from build123d import *

# Parameters (mm, degrees)
EXTRUDE_1_DEPTH     = 3
SKETCH_2_W          = 3
SKETCH_2_H          = 26
EXTRUDE_2_DEPTH     = 53.5
FILLET_1_R          = 4
FILLET_2_R          = 2
FILLET_3_R          = 1
SKETCH_3_W          = 1.7
SKETCH_3_H          = 1.7
CUT_EXTRUDE_1_DEPTH = 3
SKETCH_4_R          = 2
CUT_EXTRUDE_2_DEPTH = 1.6
SKETCH_5_W          = 1.7
SKETCH_5_H          = 1.7
CUT_EXTRUDE_3_DEPTH = 3
SKETCH_6_R          = 2
CUT_EXTRUDE_4_DEPTH = 1.6
CUT_EXTRUDE_5_DEPTH = 3


with BuildPart() as part:
    # Эскиз1 → Бобышка-Вытянуть1 (new body)
    with BuildSketch(Plane(origin=(0, 0, 0), x_dir=(1, 0, 0), z_dir=(0, 1, 0))):
        with BuildLine():
            Line((-27.082461997, 18.034885268), (36.497538003, 18.034885268))
            Line((36.497538003, 18.034885268), (36.497538003, -7.965114732))
            Line((36.497538003, -7.965114732), (-27.082461997, -7.965114732))
            ThreePointArc((-27.082461997, -7.965114732), (-29.910889121, -6.793541857), (-31.082461997, -3.965114732))
            Line((-31.082461997, -3.965114732), (-31.082461997, 14.034885268))
            ThreePointArc((-31.082461997, 14.034885268), (-29.910889121, 16.863312393), (-27.082461997, 18.034885268))
        make_face()
    extrude(amount=EXTRUDE_1_DEPTH)

    # Эскиз2 → Бобышка-Вытянуть2 (add)
    with BuildSketch(Plane(origin=(0, 3, 0), x_dir=(1, 0, 0), z_dir=(0, 1, 0))):
        with Locations((34.997538003, 5.034885268)):
            Rectangle(SKETCH_2_W, SKETCH_2_H)
    extrude(amount=EXTRUDE_2_DEPTH)

    # Скругление1
    fillet_1_edges = [part.edges().sort_by_distance(p)[0] for p in [
        (34.997538003, 56.5, -18.034885268),
        (34.997538003, 56.5, 7.965114732),
    ]]
    fillet(fillet_1_edges, radius=FILLET_1_R)

    # Скругление2
    fillet_2_edges = [part.edges().sort_by_distance(p)[0] for p in [
        (36.497538003, 0, -5.034885268),
    ]]
    fillet(fillet_2_edges, radius=FILLET_2_R)

    # Скругление3
    fillet_3_edges = [part.edges().sort_by_distance(p)[0] for p in [
        (33.497538003, 3, -5.034885268),
    ]]
    fillet(fillet_3_edges, radius=FILLET_3_R)

    # Эскиз3 → Вырез-Вытянуть1 (cut)
    with BuildSketch(Plane.XZ):
        with Locations((-5.152461997, -5.034885268)):
            Rectangle(SKETCH_3_W, SKETCH_3_H)
        with Locations((14.147538003, -5.034885268)):
            Rectangle(SKETCH_3_W, SKETCH_3_H)
    extrude(amount=-CUT_EXTRUDE_1_DEPTH, mode=Mode.SUBTRACT)

    # Эскиз4 → Вырез-Вытянуть2 (cut)
    with BuildSketch(Plane.XZ):
        with Locations((-5.152461997, -5.034885268)):
            Circle(SKETCH_4_R)
        with Locations((14.147538003, -5.034885268)):
            Circle(SKETCH_4_R)
    extrude(amount=-CUT_EXTRUDE_2_DEPTH, mode=Mode.SUBTRACT)

    # Эскиз5 → Вырез-Вытянуть3 (cut)
    with BuildSketch(Plane(origin=(36.497538003, 0, 0), x_dir=(0, 0, -1), z_dir=(1, 0, 0))):
        with Locations((5.034885268, 21.35)):
            Rectangle(SKETCH_5_W, SKETCH_5_H)
        with Locations((5.034885268, 40.65)):
            Rectangle(SKETCH_5_W, SKETCH_5_H)
    extrude(amount=-CUT_EXTRUDE_3_DEPTH, mode=Mode.SUBTRACT)

    # Эскиз6 → Вырез-Вытянуть4 (cut)
    with BuildSketch(Plane(origin=(36.497538003, 0, 0), x_dir=(0, 0, -1), z_dir=(1, 0, 0))):
        with Locations((5.034885268, 40.65)):
            Circle(SKETCH_6_R)
        with Locations((5.034885268, 21.35)):
            Circle(SKETCH_6_R)
    extrude(amount=-CUT_EXTRUDE_4_DEPTH, mode=Mode.SUBTRACT)

    # Эскиз7 → Вырез-Вытянуть5 (cut)
    with BuildSketch(Plane.XZ):
        with BuildLine():
            Line((19.957538003, 0.615114732), (26.257538003, 0.615114732))
            ThreePointArc((26.257538003, 0.615114732), (26.964644784, 0.322221513), (27.257538003, -0.384885268))
            Line((27.257538003, -0.384885268), (27.257538003, -9.684885268))
            ThreePointArc((27.257538003, -9.684885268), (26.964644784, -10.391992049), (26.257538003, -10.684885268))
            Line((26.257538003, -10.684885268), (19.957538003, -10.684885268))
            ThreePointArc((19.957538003, -10.684885268), (19.250431222, -10.391992049), (18.957538003, -9.684885268))
            Line((18.957538003, -9.684885268), (18.957538003, -0.384885268))
            ThreePointArc((18.957538003, -0.384885268), (19.250431222, 0.322221513), (19.957538003, 0.615114732))
        make_face()
    extrude(amount=-CUT_EXTRUDE_5_DEPTH, mode=Mode.SUBTRACT)


solid = part.part
Here's how the part is built. I have some questions about the finished solid (model axes, mm). A direction names the side the tool comes from. Coordinates: 2 decimals unless noted, no trailing zeros. Order: outer loops, then holes, each group sorted by start corner. A loop starts at its lowest first (then second) coordinate and runs counter-clockwise, first axis right, second up. Notation, with made-up numbers: (11.25, 21.5) - (53.25, 21.5) arc R17 cw to (53.25, 31.5) - close; hole circle Ø10 at (15, 61.25). An arc over 180 degrees is marked (long way). Use CSV: the item, a comma, the result in double quotes. Start each with the question number.
1. For faces 5 (the face through (35.7, 19.6, -6)), 6 (the face through (23, 1, 0.615)), 7 (the face through (34, 39.8, -5)), 8 (the face through (12.6, 0.8, -6.3)), which set-ups out of +Z, -Z, +X, -X, +Y, -Y let a thin tool reach every point of the face, with its end or its side?
2. Suppose I cut it at C-C on x = -12. List the corners of the cut face in (y, z) for me.
3. Please list where these lines run through material, in increasing order: line 1 (Y direction, x = -10.5, z = -8.5); line 2 (X direction, y = 23, z = -10.75); line 3 (X direction, y = 22, z = -3.5). Write a range as from..to.
4. Suppose I cut it at B-B on z = 2. List the corners of the cut face in (x, y) for me, then the cut area to 3 significant figures.
5. Suppose I cut it at A-A on y = 40.65. List the corners of the cut face in (x, z) for me, then the cut area to 3 significant figures.
6. If we mould it in two halves opening along X, with no side actions, what happens to faces 1 (the face through (1, 3, -5)), 2 (the face through (33.498, 30, -5)), 3 (the face through (14, 2, -4.185)), 4 (the face through (34.898, 42, -5))? For each: +X half, -X half, draft (parallel to the pull), parting line (faces both ways), or undercut.
7. I'm going to push flat-ended pins straight in: pin 1 (1.5 mm diameter, centred on y = 1.5, z = -6, fed in from +X); pin 2 (1.2 mm diameter, centred on y = 41, z = -4.5, fed in from +X); pin 3 (4.5 mm diameter, centred on x = 14.15, z = -5.03, fed in from +Y); pin 4 (8 mm diameter, centred on y = 24, z = -5.5, fed in from -X). Where does each tip first touch, or does it pass through?
8. Suppose I cut it at D-D on y = 5. List the corners of the cut face in (x, z) for me.
Output:
1,face 5,"+X"
1,face 6,"+Y, -Y"
1,face 7,"+X, -X"
1,face 8,"-Y"
2,outline,"(0, -18.03) - (3, -18.03) - (3, 7.97) - (0, 7.97) - close"
3,line 1,"y = 0..3"
3,line 2,"x = 33.5..36.5"
3,line 3,"x = 33.5..34.9"
4,outline,"(-31.08, 0) - (34.5, 0) arc R2 ccw to (36.5, 2) - (36.5, 56.5) - (33.5, 56.5) - (33.5, 4) arc R1 cw to (32.5, 3) - (-31.08, 3) - close"
4,area,"363 mm2"
5,outline,"(33.5, -18.03) - (36.5, -18.03) - (36.5, -7.03) - (34.9, -7.03) - (34.9, -5.88) - (33.5, -5.88) - close; (33.5, -4.18) - (34.9, -4.18) - (34.9, -3.03) - (36.5, -3.03) - (36.5, 7.97) - (33.5, 7.97) - close"
5,area,"69.2 mm2"
6,face 1,"draft"
6,face 2,"-X half"
6,face 3,"undercut"
6,face 4,"+X half"
7,pin 1,"stops at x = 36.5"
7,pin 2,"stops at x = 34.9"
7,pin 3,"stops at y = 3"
7,pin 4,"stops at x = 33.5"
8,outline,"(33.5, -18.03) - (36.5, -18.03) - (36.5, 7.97) - (33.5, 7.97) - close"
